from build123d import *

# Parameters (mm, degrees)
EXTRUDE_1_DEPTH = 30


with BuildPart() as part:
    # 草图3 → 凸台-拉伸1 (new body)
    with BuildSketch(Plane(origin=(0, 0, 0), x_dir=(1, 0, 0), z_dir=(0, 1, 0))):
        with BuildLine():
            Line((-227.985581002, 0), (-261.817326429, 0))
            Line((-261.817326429, 0), (-261.817326429, 6))
            Line((-261.817326429, 6), (-221.817326429, 6))
            ThreePointArc((-221.817326429, 6), (-151.992790501, -68.953199218), (-82.168254573, 6))
            Line((-82.168254573, 6), (-69.742383097, 6))
            ThreePointArc((-69.742383097, 6), (0, -70), (69.742383097, 6))
            Line((69.742383097, 6), (80.018614475, 6))
            ThreePointArc((80.018614475, 6), (149.760997572, -70), (219.503380668, 6))
            Line((219.503380668, 6), (259.503380668, 6))
            Line((259.503380668, 6), (259.503380668, 0))
            Line((259.503380668, 0), (225.760997572, 0))
            ThreePointArc((225.760997572, 0), (156.283347312, -75.71960746), (74.880498786, -12.996572686))
            ThreePointArc((74.880498786, -12.996572686), (-6.52234974, -75.71960746), (-76, 0))
            ThreePointArc((-76, 0), (-151.992790501, -74.953199218), (-227.985581002, 0))
        make_face()
    extrude(amount=EXTRUDE_1_DEPTH)


solid = part.part
Input: part model. Units: mm. Frame: model coordinates. A direction names the side the tool comes from. Round coordinates to 2 decimals unless told otherwise and drop trailing zeros. Order: outer loops, then holes, each group sorted by start corner. A loop starts at its lowest first (then second) coordinate and runs counter-clockwise, first axis right, second up. Notation, with made-up numbers: (21.5, 38.25) - (76.5, 38.25) arc R22 ccw to (76.5, 51.25) - close; hole circle Ø8 at (78, 43). An arc over 180 degrees is marked (long way). Use a Markdown table: item, result.
1. Section A-A on z = 63. Return the cut outline in (x, y).
Evaluation:
| item | result |
|---|---|
| outline | (-192.91, 0) - (-180.24, 0) - (-180.24, 30) - (-192.91, 30) - close; (-123.74, 0) - (-111.08, 0) - (-111.08, 30) - (-123.74, 30) - close; (-42.51, 0) - (-30.51, 0) - (-30.51, 30) - (-42.51, 30) - close; (30.51, 0) - (42.51, 0) - (42.51, 30) - (30.51, 30) - close; (107.25, 0) - (119.25, 0) - (119.25, 30) - (107.25, 30) - close; (180.27, 0) - (192.27, 0) - (192.27, 30) - (180.27, 30) - close |
2. Mould query, pull axis X, two halves, no side actions, for faces 1 (the face through (-153.601, 14.79, 68.935)), 2 (the face through (-245, 15, 0)). Classes: +X half, -X half, draft (parallel to the pull), parting line (faces both ways), or undercut.
Evaluation:
| item | result |
|---|---|
| face 1 | undercut |
| face 2 | draft |
3. First-contact query: pin 1 (8 mm diameter, centred on x = 37, y = 26.5, fed in from +Z); pin 2 (15 mm diameter, centred on x = -252.5, y = 19.5, fed in from +Z); pin 3 (4 mm diameter, centred on y = 22.5, z = 67.5, fed in from +X). Flat tips, straight axial feed; report the tip coordinate or a pass-through.
Evaluation:
| item | result |
|---|---|
| pin 1 | z = 68.46 |
| pin 2 | z = 0 |
| pin 3 | x = 188.31 |
4. Access query for faces 3 (the face through (-242, 15, -6)), 4 (the face through (243, 15, 0)). Directions: +Z, -Z, +X, -X, +Y, -Y. A direction counts if a zero-diameter tool reaches every point of the face in a straight line with its end or side. Return the directions, or none.
Evaluation:
| item | result |
|---|---|
| face 3 | -Z, +X, -X, +Y, -Y |
| face 4 | +Z, +X, +Y, -Y |
5. Material intervals for probe 1 along X at (y, z) = (7.25, 28); probe 2 along X at (y, z) = (20.25, 50.5); probe 3 along X at (y, z) = (27.5, 6), sorted ascending.
Evaluation:
| item | result |
|---|---|
| probe 1 | -222.22 to -215.68, -88.3 to -81.76, -70.65 to -64.16, 64.16 to 70.65, 79.11 to 85.6, 213.92 to 220.42 |
| probe 2 | -207.84 to -199.35, -104.63 to -96.15, -56.8 to -48.47, 48.47 to 56.8, 92.97 to 101.29, 198.24 to 206.56 |
| probe 3 | -227.67 to -221.64, -82.35 to -76.32, -75.76 to -69.74, 69.74 to 80.02, 219.5 to 225.52 |
6. Section B-B on y = 21. Return the cut outline in (x, z).
Evaluation:
| item | result |
|---|---|
| outline | (-261.82, -6) - (-221.82, -6) arc R70 cw (long way) to (-82.17, -6) - (-69.74, -6) arc R70 cw (long way) to (69.74, -6) - (80.02, -6) arc R70 cw (long way) to (219.5, -6) - (259.5, -6) - (259.5, 0) - (225.76, 0) arc R76 ccw to (74.88, 13) arc R76 ccw to (-76, 0) arc R76 ccw to (-227.99, 0) - (-261.82, 0) - close |
7. Section D-D on x = 0. Return the cut outline in (y, z), then the cut area to 3 significant figures.
Evaluation:
| item | result |
|---|---|
| outline | (0, 70) - (30, 70) - (30, 76) - (0, 76) - close |
| area | 180 mm^2 |
8. Section C-C on z = 26.5. Return the cut outline in (x, y).
Evaluation:
| item | result |
|---|---|
| outline | (-222.82, 0) - (-216.34, 0) - (-216.34, 30) - (-222.82, 30) - close; (-87.64, 0) - (-81.16, 0) - (-81.16, 30) - (-87.64, 30) - close; (-71.23, 0) - (-64.79, 0) - (-64.79, 30) - (-71.23, 30) - close; (64.79, 0) - (71.23, 0) - (71.23, 30) - (64.79, 30) - close; (78.53, 0) - (84.97, 0) - (84.97, 30) - (78.53, 30) - close; (214.55, 0) - (220.99, 0) - (220.99, 30) - (214.55, 30) - close |
